```python
from build123d import *

# Parameters (mm, degrees)
SKETCH1_W           = 22.5552
SKETCH1_H           = 12.7
BOSS_EXTRUDE1_DEPTH = 1
SKETCH2_W           = 5
SKETCH2_H           = 7.3
CUT_EXTRUDE1_DEPTH  = 1
SKETCH3_W           = 5
SKETCH3_H           = 5
CUT_EXTRUDE2_DEPTH  = 1
BOSS_EXTRUDE2_DEPTH = 1
SKETCH7_W           = 1
SKETCH7_H           = 1
CUT_EXTRUDE3_DEPTH  = 3


with BuildPart() as part:
    # Sketch1 → Boss-Extrude1 (new body)
    with BuildSketch(Plane(origin=(0, 0, 0), x_dir=(1, 0, 0), z_dir=(0, 1, 0))):
        with Locations((-28.763088774, 14.606547542)):
            Rectangle(SKETCH1_W, SKETCH1_H)
    extrude(amount=BOSS_EXTRUDE1_DEPTH)

    # Sketch2 → Cut-Extrude1 (cut)
    with BuildSketch(Plane(origin=(0, 1, 0), x_dir=(1, 0, 0), z_dir=(0, 1, 0))):
        with Locations((-37.540688774, 14.606547542)):
            Rectangle(SKETCH2_W, SKETCH2_H)
    extrude(amount=-CUT_EXTRUDE1_DEPTH, mode=Mode.SUBTRACT)

    # Sketch3 → Cut-Extrude2 (cut)
    with BuildSketch(Plane(origin=(0, 1, 0), x_dir=(1, 0, 0), z_dir=(0, 1, 0))):
        with Locations((-19.985488774, 13.756547542)):
            Rectangle(SKETCH3_W, SKETCH3_H)
    extrude(amount=-CUT_EXTRUDE2_DEPTH, mode=Mode.SUBTRACT)

    # Sketch4 → Boss-Extrude2 (add)
    with BuildSketch(Plane.XZ):
        Polygon((-40.040688774, -8.256547542), (-40.040688774, -8.756547542), (-17.985488774, -8.756547542), (-17.985488774, -10.256547542), (-17.485488774, -10.256547542), (-17.485488774, -8.256547542), align=None)
        Polygon((-17.985488774, -20.456547542), (-40.040688774, -20.456547542), (-40.040688774, -20.956547542), (-17.485488774, -20.956547542), (-17.485488774, -18.456547542), (-17.985488774, -18.456547542), align=None)
    extrude(amount=BOSS_EXTRUDE2_DEPTH)

    # Sketch7 → Cut-Extrude3 (cut)
    with BuildSketch(Plane(origin=(0, 1, 0), x_dir=(1, 0, 0), z_dir=(0, 1, 0))):
        with Locations((-37.140688774, 20.456547542)):
            Rectangle(SKETCH7_W, SKETCH7_H)
        with Locations((-37.140688774, 8.756547542)):
            Rectangle(SKETCH7_W, SKETCH7_H)
        with Locations((-19.375488774, 20.456547542)):
            Rectangle(SKETCH7_W, SKETCH7_H)
        with Locations((-19.375488774, 8.756547542)):
            Rectangle(SKETCH7_W, SKETCH7_H)
    extrude(amount=-CUT_EXTRUDE3_DEPTH, mode=Mode.SUBTRACT)


solid = part.part
```
Source: CAD feature listing. Evaluate the final solid. Frame: model axes, mm. A direction names the side the tool comes from. Give positions to 0.01 mm unless a question says otherwise; leave off trailing zeros. Order: outer loops, then holes, each group sorted by start corner. A loop starts at its lowest first (then second) coordinate and runs counter-clockwise, first axis right, second up.
(1) Section query A-A (x = -19.25). Return the cut outline in (y, z), plus the area to 3 significant figures.
(2) Contact query for flat-ended pins moving along their axis: P1, Ø0.5, axis at y = -0.5, z = -19, coming from the -X side; P2, Ø0.5, axis at y = 0.5, z = -13, coming from the +X side. Output: stop coordinate, or through.
(3) Pull-direction query (X, two-part tool) for faces 6 (the face through (-19.4, 0.5, -19.957)), 7 (the face through (-28, 0, -20.957)), 8 (the face through (-22.485, 0.5, -13.7)); classes: +X half, -X half, draft (parallel to the pull), parting line (faces both ways), or undercut.
(4) Section query D-D (z = -19.25). Return the cut outline in (x, y), plus the area to 3 significant figures.
(5) Section query B-B (y = -0.3). Return the cut outline in (x, z).
(6) Section query C-C (x = -34.5). Return the cut outline in (y, z), plus the area to 3 significant figures.
(7) Material intervals for line 1 along Z through (x, y) = (-25, -0.85); line 2 along Z through (x, y) = (-38.75, 0.75); line 3 along Y through (x, z) = (-20.5, -10.25), sorted ascending.
(8) Access query for faces 1 (the face through (-18.4, -0.5, -20.457)), 2 (the face through (-17.485, 0, -9)), 3 (the face through (-18.875, 0.2, -20.6)), 4 (the face through (-36.641, 0.2, -8.6)), 5 (the face through (-18, 0, -20.957)). Directions: +Z, -Z, +X, -X, +Y, -Y. A direction counts if a zero-diameter tool reaches every point of the face in a straight line with its end or side. Return the directions, or none.
Outcome:
1. outline: (0, -19.96) - (1, -19.96) - (1, -16.26) - (0, -16.26) - close; (0, -11.26) - (1, -11.26) - (1, -9.26) - (0, -9.26) - close
1. area: 5.70 mm2
2. P1: stops at x = -17.99
2. P2: stops at x = -22.49
3. face 6: undercut
3. face 7: draft
3. face 8: +X half
4. outline: (-40.04, 0) - (-17.99, 0) - (-17.99, -1) - (-17.49, -1) - (-17.49, 1) - (-40.04, 1) - close
4. area: 23.1 mm2
5. outline: (-40.04, -20.96) - (-37.64, -20.96) - (-37.64, -20.46) - (-40.04, -20.46) - close; (-40.04, -8.76) - (-37.64, -8.76) - (-37.64, -8.26) - (-40.04, -8.26) - close; (-36.64, -20.96) - (-19.88, -20.96) - (-19.88, -20.46) - (-36.64, -20.46) - close; (-36.64, -8.76) - (-19.88, -8.76) - (-19.88, -8.26) - (-36.64, -8.26) - close; (-18.88, -20.96) - (-17.49, -20.96) - (-17.49, -18.46) - (-17.99, -18.46) - (-17.99, -20.46) - (-18.88, -20.46) - close; (-18.88, -8.76) - (-17.99, -8.76) - (-17.99, -10.26) - (-17.49, -10.26) - (-17.49, -8.26) - (-18.88, -8.26) - close
6. outline: (-1, -20.96) - (1, -20.96) - (1, -8.26) - (-1, -8.26) - (-1, -8.76) - (0, -8.76) - (0, -20.46) - (-1, -20.46) - close
6. area: 13.7 mm2
7. line 1: z = -20.96 to -20.46, -8.76 to -8.26
7. line 2: z = -20.96 to -18.26, -10.96 to -8.26
7. line 3: y = 0 to 1
8. face 1: -X, -Y
8. face 2: +Z, -Z, +X, +Y, -Y
8. face 3: -Z, +Y, -Y
8. face 4: +Z, +Y, -Y
8. face 5: -Z, +X, -X, +Y, -Y
